Read the model definition and answer for the solid it produces. Units are mm, in the model's axes. Face numbers are marked on the shaded views. Round coordinates to 2 decimals unless told otherwise and drop trailing zeros. Order: outer loops, then holes, each group sorted by start corner. A loop starts at its lowest first (then second) coordinate and runs counter-clockwise, first axis right, second up.
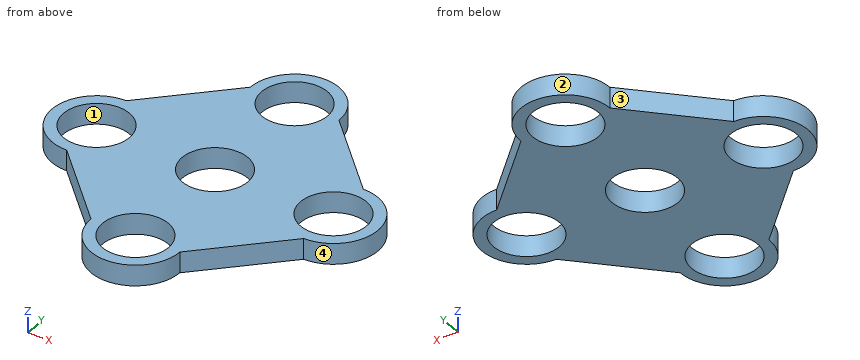
from build123d import *

# Parameters (mm, degrees)
F0_R     = 11.1
F1_DEPTH = 3.5


with BuildPart() as f1:
    # F0 (on Top) → F1 (new body, symmetric)
    with BuildSketch(Plane.XY):
        with BuildLine():
            Line((40, 15), (15, 40))
            ThreePointArc((15, 40), (0, 55), (-15, 40))
            Line((-15, 40), (-40, 15))
            ThreePointArc((-40, 15), (-55, 0), (-40, -15))
            Line((-40, -15), (-15, -40))
            ThreePointArc((-15, -40), (0, -55), (15, -40))
            Line((15, -40), (40, -15))
            ThreePointArc((40, -15), (55, 0), (40, 15))
        make_face()
        with Locations((0, -40)):
            Circle(F0_R, mode=Mode.SUBTRACT)
        with Locations((-40, 0)):
            Circle(F0_R, mode=Mode.SUBTRACT)
        Circle(F0_R, mode=Mode.SUBTRACT)
        with Locations((40, 0)):
            Circle(F0_R, mode=Mode.SUBTRACT)
        with Locations((0, 40)):
            Circle(F0_R, mode=Mode.SUBTRACT)
    extrude(amount=F1_DEPTH, both=True)


solid = f1.part
Q1. A cutting plane is placed at A-A, the plane x = 0. Give the vertices of the cut face in (y, z).
Outcome:
outline: (-55, -3.5) - (-51.1, -3.5) - (-51.1, 3.5) - (-55, 3.5) - close; (-28.9, -3.5) - (-11.1, -3.5) - (-11.1, 3.5) - (-28.9, 3.5) - close; (11.1, -3.5) - (28.9, -3.5) - (28.9, 3.5) - (11.1, 3.5) - close; (51.1, -3.5) - (55, -3.5) - (55, 3.5) - (51.1, 3.5) - close
Q2. Straight lines are drawn through the part: probe 1 along Y at (x, z) = (0, -1.5); probe 2 along Y at (x, z) = (-40, 1); probe 3 along X at (y, z) = (7, -2). For each, find the intervals that lie inside material, in ascending order.
Outcome:
probe 1: y = -55 to -51.1, -28.9 to -11.1, 11.1 to 28.9, 51.1 to 55
probe 2: y = -15 to -11.1, 11.1 to 15
probe 3: x = -53.27 to -48.61, -31.39 to -8.61, 8.61 to 31.39, 48.61 to 53.27
Q3. For a pull along X with two mould halves and no side action, classify the marked faces 1, 2, 3 and 4 as released by +X, released by -X, zero draft, split by the parting line, or undercut.
Outcome:
face 1: undercut
face 2: split by the parting line
face 3: released by -X
face 4: released by +X
Q4. A cutting plane is placed at D-D, the plane x = 45.5. Give the vertices of the cut face in (y, z), plus the area to 3 significant figures.
Outcome:
outline: (-13.96, -3.5) - (-9.64, -3.5) - (-9.64, 3.5) - (-13.96, 3.5) - close; (9.64, -3.5) - (13.96, -3.5) - (13.96, 3.5) - (9.64, 3.5) - close
area: 60.4 mm2
Q5. Flat-ended cylindrical pins translate along their axes: pin 1 (13.5 mm diameter, centred on x = 0, y = -40, fed in from -Z); pin 2 (2 mm diameter, centred on y = -38, z = 2, fed in from +X); pin 3 (3 mm diameter, centred on y = 25.5, z = -0.5, fed in from +X); pin 4 (1 mm diameter, centred on y = 31, z = 2, fed in from +X). Find the tip coordinate at first contact, or state that the pin passes through.
Outcome:
pin 1: passes through
pin 2: stops at x = 18
pin 3: stops at x = 31
pin 4: stops at x = 24.5
Q6. A cutting plane is placed at B-B, the plane z = 2. Give the vertices of the cut face in (x, y).
Outcome:
outline: (-40, -15) - (-15, -40) arc R15 ccw to (15, -40) - (40, -15) arc R15 ccw to (40, 15) - (15, 40) arc R15 ccw to (-15, 40) - (-40, 15) arc R15 ccw to start; hole circle Ø22.2 at (-40, 0); hole circle Ø22.2 at (0, -40); hole circle Ø22.2 at (0, 0); hole circle Ø22.2 at (0, 40); hole circle Ø22.2 at (40, 0)
Q7. A cutting plane is placed at C-C, the plane y = 31. Give the vertices of the cut face in (x, z), plus the area to 3 significant figures.
Outcome:
outline: (-24, -3.5) - (-6.5, -3.5) - (-6.5, 3.5) - (-24, 3.5) - close; (6.5, -3.5) - (24, -3.5) - (24, 3.5) - (6.5, 3.5) - close
area: 245 mm2
